Can you work these out from the model? Positions are in its coordinate system, mm. A direction names the side the tool comes from. Give positions to 0.01 mm unless a question says otherwise; leave off trailing zeros. Order: outer loops, then holes, each group sorted by start corner. A loop starts at its lowest first (then second) coordinate and runs counter-clockwise, first axis right, second up. Notation, with made-up numbers: M 23,49.25 L 59,49.25 A15 ccw 59,57.25 Z; hole C 81,-4.5 d6. An arc over 180 degrees is marked long. Answer as a JSON object with one key per item and string values.
```python
from build123d import *

# Parameters (mm, degrees)
SKETCH_1_W            = 30
SKETCH_1_H            = 13.5
EXTRUDE_1_DEPTH       = 20
SKETCH_2_W            = 10
SKETCH_2_H            = 20.163242361
CUT_EXTRUDE_2_DEPTH   = 29.41214529
SKETCH_3_R            = 3
CUT_EXTRUDE_3_DEPTH   = 37.827299657
SKETCH_6_W            = 30
SKETCH_6_H            = 13.5
EXTRUDE_5_DEPTH       = 10
SKETCH_7_R            = 3
CUT_EXTRUDE_1_DEPTH   = 29.41214529
SKETCH_8_W            = 30
SKETCH_8_H            = 18
CUT_EXTRUDE_2_2_DEPTH = 5
CHAMFER_1_SIZE        = 2
SKETCH_9_W            = 6.52399098
SKETCH_9_H            = 33.458140235
CUT_EXTRUDE_6_DEPTH   = 29.41214529
SKETCH_14_W           = 84.903926308
SKETCH_14_H           = 44.963333207
CUT_EXTRUDE_10_DEPTH  = 1
SKETCH_15_R           = 2.000000004
CUT_EXTRUDE_3_2_DEPTH = 16


with BuildPart() as part:
    # Эскиз1 → Вытянуть1 (new body)
    with BuildSketch(Plane.XY):
        with Locations((0, -0.75)):
            Rectangle(SKETCH_1_W, SKETCH_1_H)
    extrude(amount=EXTRUDE_1_DEPTH)

    # Эскиз2 → Cut-Extrude 2 (cut, through all)
    with BuildSketch(Plane.XZ.offset(7.5)):
        with Locations((0, 18.081621181)):
            Rectangle(SKETCH_2_W, SKETCH_2_H)
    extrude(amount=-CUT_EXTRUDE_2_DEPTH, mode=Mode.SUBTRACT)

    # Эскиз3 → Cut-Extrude 3 (cut, through all)
    with BuildSketch(Plane(origin=(15, 0, 0), x_dir=(0, 0, -1), z_dir=(1, 0, 0))):
        with Locations(Location((-14.861357689, 0, 0), (0, 0, 90))):
            Circle(SKETCH_3_R)
    extrude(amount=-CUT_EXTRUDE_3_DEPTH, mode=Mode.SUBTRACT)

    # Эскиз6 → Вытянуть5 (add)
    with BuildSketch(Plane(origin=(0, 0, 0), x_dir=(-1, 0, 0), z_dir=(0, 0, -1))):
        with Locations((0, -0.75)):
            Rectangle(SKETCH_6_W, SKETCH_6_H)
    extrude(amount=EXTRUDE_5_DEPTH)

    # Эскиз7 → Вырез-Вытянуть1 (cut, through all)
    with BuildSketch(Plane(origin=(0, 6, 0), x_dir=(1, 0, 0), z_dir=(0, 1, 0))):
        with Locations(Location((0.231400022, 0.869933179, 0), (0, 0, 270))):
            Circle(SKETCH_7_R)
    extrude(amount=-CUT_EXTRUDE_1_DEPTH, mode=Mode.SUBTRACT)

    # Эскиз8 → Cut-Extrude 2 2 (cut)
    with BuildSketch(Plane.XZ.offset(7.5)):
        with Locations((0, -1)):
            Rectangle(SKETCH_8_W, SKETCH_8_H)
    extrude(amount=-CUT_EXTRUDE_2_2_DEPTH, mode=Mode.SUBTRACT)

    # Фаска1
    chamfer_1_edges = [part.edges().sort_by_distance(p)[0] for p in [
        (-10, -7.5, 20),
        (-10, 6, 20),
        (10, -7.5, 20),
        (10, -7.5, 8),
        (-10, -7.5, 8),
        (10, 6, 20),
    ]]
    chamfer(chamfer_1_edges, length=CHAMFER_1_SIZE)

    # Эскиз9 → Вытянуть6 (cut, through all)
    with BuildSketch(Plane(origin=(0, 6, 0), x_dir=(1, 0, 0), z_dir=(0, 1, 0))):
        with Locations((16.26199549, -3.329208479)):
            Rectangle(SKETCH_9_W, SKETCH_9_H)
        with Locations((-16.26199549, -3.329208479)):
            Rectangle(SKETCH_9_W, SKETCH_9_H)
    extrude(amount=-CUT_EXTRUDE_6_DEPTH, mode=Mode.SUBTRACT)

    # Эскиз14 → Вытянуть10 (cut)
    with BuildSketch(Plane.XZ.offset(7.5)):
        with Locations((0.061866905, -0.327668242)):
            Rectangle(SKETCH_14_W, SKETCH_14_H)
    extrude(amount=-CUT_EXTRUDE_10_DEPTH, mode=Mode.SUBTRACT)

    # Эскиз15 → Cut-Extrude 3 2 (cut)
    with BuildSketch(Plane(origin=(0, 0, -10), x_dir=(-1, 0, 0), z_dir=(0, 0, -1))):
        with Locations((-7.999999896, 1.748498224)):
            Circle(SKETCH_15_R)
        with Locations((8.000000104, 1.750000003)):
            Circle(SKETCH_15_R)
    extrude(amount=-CUT_EXTRUDE_3_2_DEPTH, mode=Mode.SUBTRACT)


solid = part.part
```
1) Thinking about a two-plate mould opening in X: for faces 4 (the face through (13, 1, 5)), 5 (the face through (-9, -4, 8)), 6 (the face through (-8, 2, 6)), which applies, pulls with the +X half, pulls with the -X half, needs draft (parallel to the pull), parting line crosses it, or undercut?
Results found:
{"face 4": "pulls with the +X half", "face 5": "needs draft", "face 6": "undercut"}
2) I want a section at C-C on y = 1.25. Write out the boundary of the cut face in (x, z), and give its area (3 significant figures).
Results found:
{"outline": "M -13,-10 L -9.94,-10 L -9.94,6 L -6.06,6 L -6.06,-10 L 6.06,-10 L 6.06,6 L 9.94,6 L 9.94,-10 L 13,-10 L 13,12.13 L 5,12.13 L 5,8 L -5,8 L -5,12.13 L -13,12.13 Z; M -13,17.59 L -5,17.59 L -5,20 L -13,20 Z; M 5,17.59 L 13,17.59 L 13,20 L 5,20 Z; hole C 0.23,-0.87 d6", "area": "421 mm²"}
3) I'm going to push flat-ended pins straight in: pin 1 Ø7 at (x, y) = (1, 2.5) entering from +Z; pin 2 Ø3 at (x, y) = (-8, 1.75) entering from -Z; pin 3 Ø3 at (x, z) = (-7, 6) entering from -Y. Where does each tip first touch, or does it pass through?
Results found:
{"pin 1": "stops at z = 8", "pin 2": "stops at z = 6", "pin 3": "stops at y = -2.5"}
4) I want a section at B-B on z = 0. Write out the boundary of the cut face in (x, y).
Results found:
{"outline": "M -13,-2.5 L -2.64,-2.5 L -2.64,6 L -13,6 Z; M 3.1,-2.5 L 13,-2.5 L 13,6 L 3.1,6 Z; hole C -8,1.75 d4; hole C 8,1.75 d4"}
5) I need wall thicknesses on L1, parallel to Y at x = -8, z = -3.75; L2, parallel to X at y = 4.25, z = 8.5; L3, parallel to X at y = 3.5, z = -5.25. Which ranges of each line are inside material? Lowest first, please.
Results found:
{"L1": "y = -2.5 to -0.25, 3.75 to 6", "L2": "x = -13 to -5, 5 to 13", "L3": "x = -13 to -8.97, -7.03 to 7.03, 8.97 to 13"}
6) I want a section at A-A on y = -3.5. Write out the boundary of the cut face in (x, z), and give its area (3 significant figures).
Results found:
{"outline": "M -13,8 L -5,8 L -5,20 L -13,20 Z; M 5,8 L 13,8 L 13,20 L 5,20 Z", "area": "192 mm²"}
7) For faces 1 (the face through (-9, 5, 19)), 2 (the face through (0, 2, 8)), 3 (the face through (8, 2, 6)), which set-ups out of +Z, -Z, +X, -X, +Y, -Y let a thin tool reach every point of the face, with its end or its side?
Results found:
{"face 1": "+Z, +X, -X, +Y", "face 2": "+Z, +Y, -Y", "face 3": "-Z"}
8) I want a section at D-D on z = 10.25. Write out the boundary of the cut face in (x, y), and give its area (3 significant figures).
Results found:
{"outline": "M -13,-6.5 L -5,-6.5 L -5,6 L -13,6 Z; M 5,-6.5 L 13,-6.5 L 13,6 L 5,6 Z", "area": "200 mm²"}
